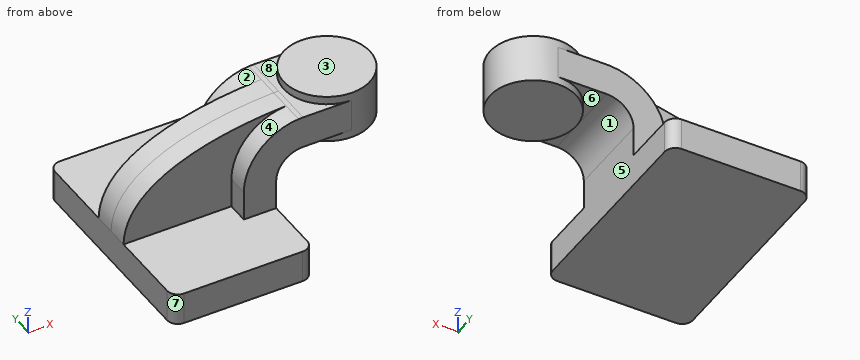
from build123d import *

# Parameters (mm, degrees)
F1_DEPTH = 63.5
F0_W     = 25.4
F0_H     = 19.05
F2_DEPTH = 25.4
F3_DEPTH = 12.7
F5_R     = 6.35


with BuildPart() as f1:
    # F0 (on Front) → F1 (new body, symmetric)
    with BuildSketch(Plane.XZ):
        Polygon((41.275, -9.525), (41.275, 9.525), (22.225, 9.525), (-41.275, 9.525), (-41.275, -9.525), align=None)
    extrude(amount=F1_DEPTH, both=True)

    # F0 (on Front) → F2 (join, symmetric)
    with BuildSketch(Plane.XZ):
        with BuildLine():
            Line((22.225, 9.525), (41.275, 9.525))
            Line((41.275, 9.525), (41.275, 27.0002))
            ThreePointArc((41.275, 27.0002), (45.9246798487, 38.2255201513), (57.15, 42.8752))
            Line((57.15, 42.8752), (60.325, 42.8752))
            Line((60.325, 42.8752), (60.325, 61.9252))
            Line((60.325, 61.9252), (57.15, 61.9252))
            add(Edge.make_bspline(
                [(57.15, 61.9252), (56.2667077822, 61.896021647), (55.3761352592, 61.8619828638), (54.478998675, 61.8229135204)],
                knots=[0, 0, 0, 0, 2.4041331296, 2.4041331296, 2.4041331296, 2.4041331296], degree=3))
            ThreePointArc((54.478998675, 61.8229135204), (31.527350388, 50.7327820732), (22.225, 27.0002))
            Line((22.225, 27.0002), (22.225, 9.525))
        make_face()
        with Locations((73.025, 52.4002)):
            Rectangle(F0_W, F0_H)
    extrude(amount=F2_DEPTH, both=True)

    # F0 (on Front) → F3 (join, symmetric)
    with BuildSketch(Plane.XZ):
        with BuildLine():
            Line((-41.275, 9.525), (22.225, 9.525))
            Line((22.225, 9.525), (22.225, 27.0002))
            ThreePointArc((22.225, 27.0002), (31.527350388, 50.7327820732), (54.478998675, 61.8229135204))
            add(Edge.make_bspline(
                [(54.478998675, 61.8229135204), (13.7666264229, 60.0499330393), (-40.4636171483, 47.9171368139), (-41.275, 9.525)],
                knots=[2.4041331296, 2.4041331296, 2.4041331296, 2.4041331296, 111.5045361635, 111.5045361635, 111.5045361635, 111.5045361635], degree=3))
        make_face()
    extrude(amount=F3_DEPTH, both=True)

    # F0 (on Front) → F4 (revolve)
    with BuildSketch(Plane.XZ):
        Polygon((85.725, 61.9252), (85.725, 42.8752), (85.725, 38.1), (111.125, 38.1), (111.125, 66.675), (85.725, 66.675), align=None)
    revolve(axis=Axis((85.725, 0, 52.3875), (0, 0, -1)))

    # F5
    f5_edges = [f1.edges().sort_by_distance(p)[0] for p in [
        (-41.275, -63.5, 0),
        (41.275, -63.5, 0),
        (41.275, 63.5, 0),
        (-41.275, 63.5, 0),
    ]]
    fillet(f5_edges, radius=F5_R)


solid = f1.part
Can you work these out from the model? Positions are in its coordinate system, mm. Face numbers are marked on the shaded views. A direction names the side the tool comes from. Coordinates: 2 decimals unless noted, no trailing zeros. Write each loop counter-clockwise with the first axis right and the second up, starting at its lowest first coordinate (ties: lowest second). Pieces come first, ordered by that corner, then holes. Notation, with made-up numbers: (-13, 87.25) -> (10, 87.25) arc R33 cw to (10, 125.25) -> close; hole circle Ø4 at (42, 14). An arc over 180 degrees is marked (long way). Write item = value, one per line.
(1) For pin 1 (14 mm diameter, centred on y = 19, z = 22.5, fed in from -X); pin 2 (15.5 mm diameter, centred on x = 23.5, z = 38.5, fed in from +Y); pin 3 (1 mm diameter, centred on y = -5.5, z = 49, fed in from -X), each with a flat end and sliding along its axis, tell me the tip position at first contact or that it passes through.
Verdict:
pin_1 = -39.75
pin_2 = 25.4
pin_3 = -10.41
(2) If I drill on probe 1 along Z at (x, y) = (11.5, 19.5) (3 decimals); probe 2 along Y at (x, z) = (-19, 34); probe 3 along X at (y, z) = (-20.5, 23) (3 decimals), over which ranges is the centre line in solid material (lowest first)?
Verdict:
probe_1 = -9.525 to 9.525
probe_2 = -12.7 to 12.7
probe_3 = 22.225 to 41.275
(3) On a 3-axis mill with a long thin cutter (end or side, diameter ignored), from which of +Z, -Z, +X, -X, +Y, -Y can I reach the whole of each face in a straight line? I mean the marked faces 1, 2, 3, 4 and 5. Say none if no direction works.
Verdict:
face_1 = -Z, +Y, -Y
face_2 = +Z, -X, +Y
face_3 = +Z, +X, -X, +Y, -Y
face_4 = +Z, -X, -Y
face_5 = -Z, +X, +Y, -Y
(4) Imagine slicing it at A-A (y = 38). Please give me the cut outline in (x, z) (3 decimals), and give its area (3 significant figures).
Verdict:
outline = (-41.275, -9.525) -> (41.275, -9.525) -> (41.275, 9.525) -> (-41.275, 9.525) -> close
area = 1,570 mm^2
(5) Thinking about a two-plate mould opening in X: for the marked faces 6, 7 and 8, which applies, +X half, -X half, draft (parallel to the pull), parting line (faces both ways), or undercut?
Verdict:
face_6 = undercut
face_7 = -X half
face_8 = draft
